```python
from build123d import *

# Parameters (mm, degrees)
BOSS_EXTRUDE1_DEPTH = 6.5


with BuildPart() as part:
    # Sketch1 → Boss-Extrude1 (new body)
    with BuildSketch(Plane.XY):
        with BuildLine():
            Line((6.335498205, 3.847751906), (0, 7.505553499))
            Line((0, 7.505553499), (-6.4, 3.810511777))
            Line((-6.4, 3.810511777), (-6.4, 12.338962679))
            ThreePointArc((-6.4, 12.338962679), (-0.036282053, 13.899952648), (6.335498205, 12.37220524))
            Line((6.335498205, 12.37220524), (6.335498205, 3.847751906))
        make_face()
    extrude(amount=BOSS_EXTRUDE1_DEPTH)


solid = part.part
```
Read the model definition and answer for the solid it produces. Units are mm, in the model's axes. A direction names the side the tool comes from. Coordinates: 2 decimals unless noted, no trailing zeros. Loops run counter-clockwise (first coordinate to the right, second up) from the corner with the lowest first, then second, coordinate; pieces in that order, holes last.
(1) The part is cut by section B-B (z = 4.75). Determine the outline of the cut face in (x, y).
Solution:
outline: (-6.4, 3.81) - (0, 7.51) - (6.34, 3.85) - (6.34, 12.37) arc R13.9 ccw to (-6.4, 12.34) - close
(2) A tool of negligible diameter and unlimited length cuts with its end or side. For faces 4 (the face through (-0.1, 13.9, 3.2)), 5 (the face through (3.21, 5.65, 3.2)), from which of +Z, -Z, +X, -X, +Y, -Y can it reach the whole face along a straight path? Write none if from no direction.
Solution:
face 4: +Z, -Z, +Y
face 5: +Z, -Z, -Y
(3) The part is cut by section C-C (x = -4.25). Determine the outline of the cut face in (y, z), and give its area (3 significant figures).
Solution:
outline: (5.05, 0) - (13.23, 0) - (13.23, 6.5) - (5.05, 6.5) - close
area: 53.2 mm2
(4) The part is cut by section A-A (y = 6.25). Determine the outline of the cut face in (x, z).
Solution:
outline: (-6.4, 0) - (-2.17, 0) - (-2.17, 6.5) - (-6.4, 6.5) - close; (2.17, 0) - (6.34, 0) - (6.34, 6.5) - (2.17, 6.5) - close
(5) Consider line 1 along X through (y, z) = (5, 5); line 2 along X through (y, z) = (7, 3.5); line 3 along Y through (x, z) = (-4.75, 4.25). Determine where each line is inside the solid, lowest interval first.
Solution:
line 1: x = -6.4 to -4.34, 4.34 to 6.34
line 2: x = -6.4 to -0.88, 0.88 to 6.34
line 3: y = 4.76 to 13.06
(6) The part is cut by section D-D (y = 12.75). Determine the outline of the cut face in (x, z).
Solution:
outline: (-5.54, 0) - (5.54, 0) - (5.54, 6.5) - (-5.54, 6.5) - close
(7) The mould has two halves that part along X. Classify faces 1 (the face through (6.335, 8, 3)), 2 (the face through (-3.16, 5.68, 3.2)), 3 (the face through (0, 9, 6.5)): released by +X, released by -X, zero draft, split by the parting line, or undercut.
Solution:
face 1: released by +X
face 2: undercut
face 3: zero draft
